Input: part model. Units: mm. Frame: model coordinates. A direction names the side the tool comes from. Give positions to 0.01 mm unless a question says otherwise; leave off trailing zeros. Loops run counter-clockwise (first coordinate to the right, second up) from the corner with the lowest first, then second, coordinate; pieces in that order, holes last. Notation, with made-up numbers: (70.25, 85.5) -> (93.25, 85.5) arc R27 cw to (93.25, 123.5) -> close; hole circle Ø6 at (1.25, 74.25). An arc over 180 degrees is marked (long way). Answer in a Markdown table with one row per item. Add a question column.
Autodesk Inventor part; units mm, degrees
ref_plane "bolt_to_nut_XY" through (45, 0, 0) normal (1, 0, 0) x (0, 0, -1)
ref_plane "bolt_to_nut_YZ" through (45, 0, 0) normal (0, 0, -1) x (0, 1, 0)
ref_plane "bolt_to_nut_ZX" through (45, 0, 0) normal (0, 1, 0) x (1, 0, 0)
sketch "Sketch_2" plane through (0, 0, 0) normal (0, 0, 1) x (1, 0, 0)
  line L0 (45, 0) -> (-5, 0)
  line L1 (-5, 0) -> (-5, 3.75)
  line L2 (-5, 3.75) -> (-4.5, 4.25)
  line L3 (-4.5, 4.25) -> (0, 4.25)
  line L4 (0, 4.25) -> (0, 2.5)
  line L5 (0, 2.5) -> (44.5095, 2.5)
  line L6 (44.5095, 2.5) -> (45, 2.0095)
  line L7 (45, 2.0095) -> (45, 0)
  line L8 (45, 0) -> (-5, 0)
revolve "Revolution1" add sketch "Sketch_2" angle 360 about axis through (45, 0, 0) along (1, 0, 0)
thread "Thread1"
sketch "Sketch2" plane through (-5, 0, 0) normal (-1, 0, 0) x (0, 0, 1)
  point P0 (0, 0)
hole "Hole1" at (-5, 0, 0) direction (1, 0, 0) diameter 4 depth 2.5 tip angle 150
sketch "Sketch_3" plane through (-5, 0, 0) normal (1, 0, 0) x (0, 0, -1)
  line L0 (-2, -1.1547) -> (0, -2.3094)
  line L1 (0, -2.3094) -> (2, -1.1547)
  line L2 (2, -1.1547) -> (2, 1.1547)
  line L3 (2, 1.1547) -> (0, 2.3094)
  line L4 (0, 2.3094) -> (-2, 1.1547)
  line L5 (-2, 1.1547) -> (-2, -1.1547)
extrude "Extrusion1" cut sketch "Sketch_3" along normal blind 2.5
ref_plane "bolt_to_nut_XY" through (45, 0, 0) normal (1, 0, 0) x (0, 0, -1)
ref_plane "bolt_to_nut_YZ" through (45, 0, 0) normal (0, 0, -1) x (0, 1, 0)
ref_plane "bolt_to_nut_ZX" through (45, 0, 0) normal (0, 1, 0) x (1, 0, 0)
ref_plane "screw1_XY" through (0, 0, 0) normal (1, 0, 0) x (0, 0, -1)
ref_plane "screw1_YZ" through (0, 0, 0) normal (0, 0, -1) x (0, 1, 0)
ref_plane "screw1_ZX" through (0, 0, 0) normal (0, 1, 0) x (1, 0, 0)
properties part number "CB5-45" material "鋼、炭素鋼"
1) Pull-direction query (Z, two-part tool) for faces 1 (the face through (45, 0, 0)), 2 (the face through (-1.998, -0.122, -0.027)), 3 (the face through (-2.218, 2.285, 3.584)), 4 (the face through (-4, 0, 2)); classes: +Z half, -Z half, draft (parallel to the pull), parting line (faces both ways), or undercut.
2) Reachability of faces 5 (the face through (-3.77, 1.74, 0.99)), 6 (the face through (0, 2, -2)), 7 (the face through (-5, 2, -2)) from +Z, -Z, +X, -X, +Y, -Y: full face, straight path, thin tool, end or side. Return the list, or none.
3) Material intervals for line 1 along X through (y, z) = (-2, 3); line 2 along Y through (x, z) = (24.5, -1.5); line 3 along Y through (x, z) = (-3, 3.25), sorted ascending.
4) Pin query (flat end, axial travel): pin 1 (1 mm diameter, centred on x = 1.5, z = -2, fed in from -Y); pin 2 (1.5 mm diameter, centred on y = -2, z = -2.5, fed in from +X); pin 3 (2 mm diameter, centred on x = 28, y = 2.5, fed in from -Z). Return the tip coordinate at first contact, or that it passes through.
5) Section A-A on x = 5.5. Output: boundary loops of the cut face in (y, z), and give its area (3 significant figures).
Working result:
| question | item | result |
|---|---|---|
| 1 | face 1 | draft |
| 1 | face 2 | undercut |
| 1 | face 3 | parting line |
| 1 | face 4 | undercut |
| 2 | face 5 | -X |
| 2 | face 6 | +X |
| 2 | face 7 | +Z, -Z, -X, +Y, -Y |
| 3 | line 1 | x = -5 to 0 |
| 3 | line 2 | y = -2 to 2 |
| 3 | line 3 | y = -2.74 to 2.74 |
| 4 | pin 1 | stops at y = -2 |
| 4 | pin 2 | stops at x = 44.56 |
| 4 | pin 3 | stops at z = -2 |
| 5 | outline | circle Ø5 at (0, 0) |
| 5 | area | 19.6 mm2 |
